Source: CAD feature listing. Evaluate the final solid. Frame: model axes, mm. Coordinates: 2 decimals unless noted, no trailing zeros. Order: outer loops, then holes, each group sorted by start corner. A loop starts at its lowest first (then second) coordinate and runs counter-clockwise, first axis right, second up. Notation, with made-up numbers: (29.5, -39.5) -> (37.5, -39.5) arc R18 ccw to (37.5, -5.5) -> close; hole circle Ø11 at (7, 17.25). An arc over 180 degrees is marked (long way). Write item = value, one per line. Start each with the question number.
Item 1: Section query B-B (x = 0). Output: boundary loops of the cut face in (y, z).
Item 2: Section query A-A (z = 0). Output: boundary loops of the cut face in (x, y), then the cut area to 4 significant figures.
Item 3: Contact query for flat-ended pins moving along their axis: pin 1 (3 mm diameter, centred on x = -46.5, y = 3, fed in from +Z); pin 2 (3 mm diameter, centred on x = 62, y = 7, fed in from +Z); pin 3 (4 mm diameter, centred on y = 5.5, z = 62.5, fed in from -X). Output: stop coordinate, or through.
Item 4: Ray query, line 1 along Z through (x, y) = (0, 0.2); line 2 along X through (y, z) = (7.8, 0); line 3 along X through (y, z) = (4.75, 0). Return the intervals inside material, ascending. Write a range as [from, to].
Item 5: Section query C-C (y = 3). Output: boundary loops of the cut face in (x, z), then the cut area to 3 significant figures.
```python
from build123d import *

# Parameters (mm, degrees)
SKETCH_1_R          = 83
SKETCH_1_R_2        = 75
EXTRUDE_1_DEPTH     = 8
SKETCH_2_R          = 80
SKETCH_2_R_2        = 77
CUT_EXTRUDE_1_DEPTH = 0.5
SKETCH_3_R          = 79.5
SKETCH_3_R_2        = 77
CUT_EXTRUDE_2_DEPTH = 0.5


with BuildPart() as part:
    # 草图1 → 凸台-拉伸1 (new body)
    with BuildSketch(Plane(origin=(0, 0, 0), x_dir=(1, 0, 0), z_dir=(0, 1, 0))):
        Circle(SKETCH_1_R)
        Circle(SKETCH_1_R_2, mode=Mode.SUBTRACT)
    extrude(amount=EXTRUDE_1_DEPTH)

    # 草图2 → 切除-拉伸1 (cut)
    with BuildSketch(Plane(origin=(0, 8, 0), x_dir=(1, 0, 0), z_dir=(0, 1, 0))):
        Circle(SKETCH_2_R)
        Circle(SKETCH_2_R_2, mode=Mode.SUBTRACT)
    extrude(amount=-CUT_EXTRUDE_1_DEPTH, mode=Mode.SUBTRACT)

    # 草图3 → 切除-拉伸2 (cut)
    with BuildSketch(Plane.XZ):
        Circle(SKETCH_3_R)
        Circle(SKETCH_3_R_2, mode=Mode.SUBTRACT)
    extrude(amount=-CUT_EXTRUDE_2_DEPTH, mode=Mode.SUBTRACT)


solid = part.part
```
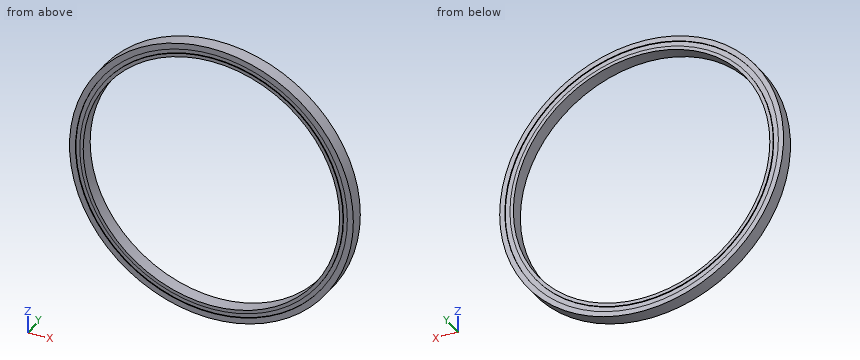
Computed:
q1.outline = (0, -83) -> (8, -83) -> (8, -80) -> (7.5, -80) -> (7.5, -77) -> (8, -77) -> (8, -75) -> (0, -75) -> (0, -77) -> (0.5, -77) -> (0.5, -79.5) -> (0, -79.5) -> close; (0, 75) -> (8, 75) -> (8, 77) -> (7.5, 77) -> (7.5, 80) -> (8, 80) -> (8, 83) -> (0, 83) -> (0, 79.5) -> (0.5, 79.5) -> (0.5, 77) -> (0, 77) -> close
q2.outline = (-83, 0) -> (-79.5, 0) -> (-79.5, 0.5) -> (-77, 0.5) -> (-77, 0) -> (-75, 0) -> (-75, 8) -> (-77, 8) -> (-77, 7.5) -> (-80, 7.5) -> (-80, 8) -> (-83, 8) -> close; (75, 0) -> (77, 0) -> (77, 0.5) -> (79.5, 0.5) -> (79.5, 0) -> (83, 0) -> (83, 8) -> (80, 8) -> (80, 7.5) -> (77, 7.5) -> (77, 8) -> (75, 8) -> close
q2.area = 122.5 mm^2
q3.pin_1 = 69.74
q3.pin_2 = 56.82
q3.pin_3 = -56.82
q4.line_1 = [-83, -79.5], [-77, -75], [75, 77], [79.5, 83]
q4.line_2 = [-83, -80], [-77, -75], [75, 77], [80, 83]
q4.line_3 = [-83, -75], [75, 83]
q5.outline = circle Ø166 at (0, 0); hole circle Ø150 at (0, 0)
q5.area = 3,970 mm^2
